Source: CAD feature listing. Evaluate the final solid. Frame: model axes, mm. Round coordinates to 2 decimals unless told otherwise and drop trailing zeros. Write each loop counter-clockwise with the first axis right and the second up, starting at its lowest first coordinate (ties: lowest second). Pieces come first, ordered by that corner, then holes.
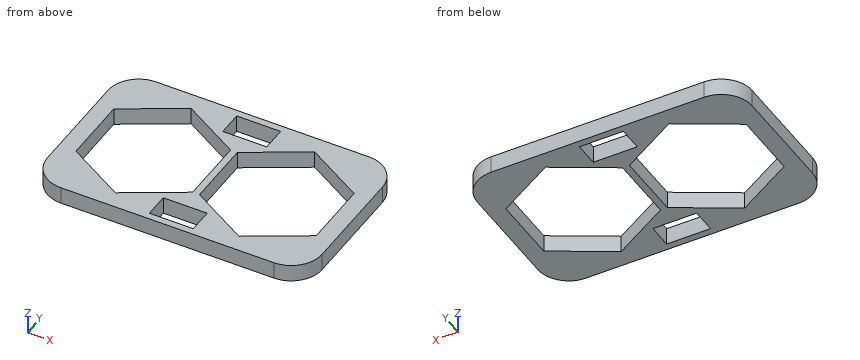
from build123d import *

# Parameters (mm, degrees)
SKETCH1_W           = 8.128
SKETCH1_H           = 4.572
BOSS_EXTRUDE1_DEPTH = 3.175


with BuildPart() as part:
    # Sketch1 → Boss-Extrude1 (new body)
    with BuildSketch(Plane.XY):
        with BuildLine():
            Line((-8.255, 15.639992312), (31.115, 15.639992312))
            ThreePointArc((31.115, 15.639992312), (35.156115254, 13.966107566), (36.83, 9.924992312))
            Line((36.83, 9.924992312), (36.83, -9.924992312))
            ThreePointArc((36.83, -9.924992312), (35.156115254, -13.966107566), (31.115, -15.639992312))
            Line((31.115, -15.639992312), (-8.255, -15.639992312))
            ThreePointArc((-8.255, -15.639992312), (-12.296115254, -13.966107566), (-13.97, -9.924992312))
            Line((-13.97, -9.924992312), (-13.97, 9.924992312))
            ThreePointArc((-13.97, 9.924992312), (-12.296115254, 13.966107566), (-8.255, 15.639992312))
        make_face()
        Polygon((12.065, -6.232496156), (22.86, -12.464992312), (33.655, -6.232496156), (33.655, 6.232496156), (22.86, 12.464992312), (12.065, 6.232496156), align=None, mode=Mode.SUBTRACT)
        Polygon((-10.795, -6.232496156), (0, -12.464992312), (10.795, -6.232496156), (10.795, 6.232496156), (0, 12.464992312), (-10.795, 6.232496156), align=None, mode=Mode.SUBTRACT)
        with Locations((11.43, 12.083992312)):
            Rectangle(SKETCH1_W, SKETCH1_H, mode=Mode.SUBTRACT)
        with Locations((11.43, -12.083992312)):
            Rectangle(SKETCH1_W, SKETCH1_H, mode=Mode.SUBTRACT)
    extrude(amount=BOSS_EXTRUDE1_DEPTH)


solid = part.part
1) Section query B-B on x = 22. Return the cut outline in (y, z) (3 decimals).
Taken from the geometry:
outline: (-15.64, 0) - (-11.968, 0) - (-11.968, 3.175) - (-15.64, 3.175) - close; (11.968, 0) - (15.64, 0) - (15.64, 3.175) - (11.968, 3.175) - close
2) Contact query for flat-ended pins moving along their axis: P1, Ø1, axis at y = 12.5, z = 2, coming from the +X side; P2, Ø3, axis at x = 17.5, y = -6.5, coming from the +Z side. Output: stop coordinate, or through.
Taken from the geometry:
P1: stops at x = 36.44
P2: passes through
3) Section query A-A on y = -5.5. Return the cut outline in (x, z) (3 decimals).
Taken from the geometry:
outline: (-13.97, 0) - (-10.795, 0) - (-10.795, 3.175) - (-13.97, 3.175) - close; (10.795, 0) - (12.065, 0) - (12.065, 3.175) - (10.795, 3.175) - close; (33.655, 0) - (36.83, 0) - (36.83, 3.175) - (33.655, 3.175) - close
4) Section query C-C on z = 0.8. Return the cut outline in (x, y) (1 decimal), then the cut area to 3 significant figures.
Taken from the geometry:
outline: (-14, -9.9) arc R5.7 ccw to (-8.3, -15.6) - (31.1, -15.6) arc R5.7 ccw to (36.8, -9.9) - (36.8, 9.9) arc R5.7 ccw to (31.1, 15.6) - (-8.3, 15.6) arc R5.7 ccw to (-14, 9.9) - close; hole (-10.8, -6.2) - (0, -12.5) - (10.8, -6.2) - (10.8, 6.2) - (0, 12.5) - (-10.8, 6.2) - close; hole (7.4, -14.4) - (15.5, -14.4) - (15.5, -9.8) - (7.4, -9.8) - close; hole (7.4, 9.8) - (15.5, 9.8) - (15.5, 14.4) - (7.4, 14.4) - close; hole (12.1, -6.2) - (22.9, -12.5) - (33.7, -6.2) - (33.7, 6.2) - (22.9, 12.5) - (12.1, 6.2) - close
area: 679 mm2
5) Section query D-D on y = 11.5. Return the cut outline in (x, z) (3 decimals), then the cut area to 3 significant figures.
Taken from the geometry:
outline: (-13.749, 0) - (-1.671, 0) - (-1.671, 3.175) - (-13.749, 3.175) - close; (1.671, 0) - (7.366, 0) - (7.366, 3.175) - (1.671, 3.175) - close; (15.494, 0) - (21.189, 0) - (21.189, 3.175) - (15.494, 3.175) - close; (24.531, 0) - (36.609, 0) - (36.609, 3.175) - (24.531, 3.175) - close
area: 113 mm2
6) Material intervals for line 1 (X direction, y = -2, z = 0.8) (3 decimals); line 2 (Y direction, x = 0, z = 2.3) (3 decimals); line 3 (X direction, y = -8.5, z = 2.45), sorted ascending.
Taken from the geometry:
line 1: x = -13.97 to -10.795, 10.795 to 12.065, 33.655 to 36.83
line 2: y = -15.64 to -12.465, 12.465 to 15.64
line 3: x = -13.97 to -6.87, 6.87 to 15.99, 29.73 to 36.83
